CAD build for the part. Positions are in the model's coordinates, mm. Face numbers are marked on the shaded views. Round coordinates to 2 decimals unless told otherwise and drop trailing zeros. Order: outer loops, then holes, each group sorted by start corner. A loop starts at its lowest first (then second) coordinate and runs counter-clockwise, first axis right, second up.
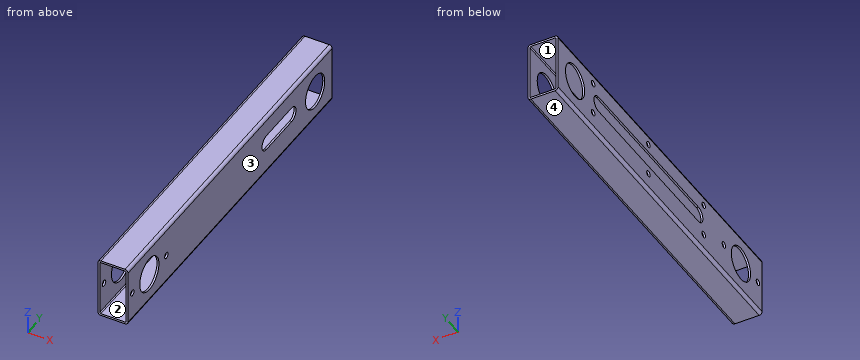
```python
from build123d import *

# Parameters (mm, degrees)
EXTRUDE_THIN1_DEPTH      = 222.25
EXTRUDE_THIN1_DEPTH_BACK = 82.55
CUT_EXTRUDE1_REACH       = 227.134
CUT_EXTRUDE4_REACH       = 227.134
SKETCH4_R                = 2.5527
CUT_EXTRUDE3_DEPTH       = 1.651
SKETCH6_R                = 14.3256
CUT_EXTRUDE5_DEPTH       = 226.134143346
F_10_CLEARANCE_HOLE1_D   = 5.1054


with BuildPart() as part:
    # Sketch1 → Extrude-Thin1 (new, two sides: drawn at the far end of the back side and taken through both)
    with BuildSketch(Plane(origin=(0, 0, 0), x_dir=(1, 0, 0), z_dir=(0, 1, 0)).offset(-EXTRUDE_THIN1_DEPTH_BACK)):
        with BuildLine():
            Line((-10.16, 25.4), (10.16, 25.4))
            ThreePointArc((10.16, 25.4), (11.956051224, 24.656051224), (12.7, 22.86))
            Line((12.7, 22.86), (12.7, -22.86))
            ThreePointArc((12.7, -22.86), (11.956051224, -24.656051224), (10.16, -25.4))
            Line((10.16, -25.4), (-10.16, -25.4))
            ThreePointArc((-10.16, -25.4), (-11.956051224, -24.656051224), (-12.7, -22.86))
            Line((-12.7, -22.86), (-12.7, 22.86))
            ThreePointArc((-12.7, 22.86), (-11.956051224, 24.656051224), (-10.16, 25.4))
        make_face()
        with BuildLine():
            Line((-10.16, 23.749), (10.16, 23.749))
            ThreePointArc((10.16, 23.749), (10.788617928, 23.488617928), (11.049, 22.86))
            Line((11.049, 22.86), (11.049, -22.86))
            ThreePointArc((11.049, -22.86), (10.788617928, -23.488617928), (10.16, -23.749))
            Line((10.16, -23.749), (-10.16, -23.749))
            ThreePointArc((-10.16, -23.749), (-10.788617928, -23.488617928), (-11.049, -22.86))
            Line((-11.049, -22.86), (-11.049, 22.86))
            ThreePointArc((-11.049, 22.86), (-10.788617928, 23.488617928), (-10.16, 23.749))
        make_face(mode=Mode.SUBTRACT)
    extrude(amount=EXTRUDE_THIN1_DEPTH + EXTRUDE_THIN1_DEPTH_BACK)

    # Sketch2 → Cut-Extrude1 (cut, up to next)
    with BuildSketch(Plane.ZY.offset(12.7), mode=Mode.PRIVATE) as cut_extrude1_sk1:
        with BuildLine():
            Line((9.2075, 161.942613489), (9.2075, 12.7))
            ThreePointArc((9.2075, 12.7), (2.54, 6.0325), (-4.1275, 12.7))
            Line((-4.1275, 12.7), (-4.1275, 161.942613489))
            ThreePointArc((-4.1275, 161.942613489), (2.54, 168.610113489), (9.2075, 161.942613489))
        make_face()
    cut_extrude1_tool1 = extrude(cut_extrude1_sk1.sketch, amount=-CUT_EXTRUDE1_REACH, mode=Mode.PRIVATE) & part.part
    add(cut_extrude1_tool1.solids().sort_by_distance((-12.7, 87.321307, 2.54))[0], mode=Mode.SUBTRACT)

    # Sketch5 → Cut-Extrude4 (cut, up to next)
    with BuildSketch(Plane(origin=(12.7, 0, 0), x_dir=(0, 0, -1), z_dir=(1, 0, 0)), mode=Mode.PRIVATE) as cut_extrude4_sk1:
        with BuildLine():
            Line((3.81, 161.942613489), (3.81, 123.842613489))
            ThreePointArc((3.81, 123.842613489), (-2.54, 117.492613489), (-8.89, 123.842613489))
            Line((-8.89, 123.842613489), (-8.89, 161.942613489))
            ThreePointArc((-8.89, 161.942613489), (-2.54, 168.292613489), (3.81, 161.942613489))
        make_face()
    cut_extrude4_tool1 = extrude(cut_extrude4_sk1.sketch, amount=-CUT_EXTRUDE4_REACH, mode=Mode.PRIVATE) & part.part
    add(cut_extrude4_tool1.solids().sort_by_distance((12.7, 142.892613, 2.54))[0], mode=Mode.SUBTRACT)

    # Sketch4 → Cut-Extrude3 (cut)
    with BuildSketch(Plane(origin=(-12.7, 0, 0), x_dir=(0, 0, -1), z_dir=(1, 0, 0))):
        with Locations(Location((11.049, 4.771306688, 0), (0, 0, 180))):
            Circle(SKETCH4_R)
        with Locations(Location((-16.129, 4.771306688, 0), (0, 0, 180))):
            Circle(SKETCH4_R)
        with Locations(Location((-16.129, 87.321306688, 0), (0, 0, 180))):
            Circle(SKETCH4_R)
        with Locations(Location((11.049, 87.321306688, 0), (0, 0, 180))):
            Circle(SKETCH4_R)
        with Locations(Location((-16.129, 169.871306688, 0), (0, 0, 180))):
            Circle(SKETCH4_R)
        with Locations(Location((11.049, 169.871306688, 0), (0, 0, 180))):
            Circle(SKETCH4_R)
    extrude(amount=CUT_EXTRUDE3_DEPTH, mode=Mode.SUBTRACT)

    # Sketch6 → Cut-Extrude5 (cut, through all)
    with BuildSketch(Plane(origin=(12.7, 0, 0), x_dir=(0, 0, -1), z_dir=(1, 0, 0))):
        with Locations((0, -50.8)):
            Circle(SKETCH6_R)
        with Locations((0, 196.85)):
            Circle(SKETCH6_R)
    extrude(amount=-CUT_EXTRUDE5_DEPTH, mode=Mode.SUBTRACT)

    # #10 Clearance Hole1 (through all)
    with Locations(Plane(origin=(12.7, 0, 0), x_dir=(0, 0, -1), z_dir=(1, 0, 0))):
        with Locations((0, -25.4), (0, -76.2)):
            Hole(F_10_CLEARANCE_HOLE1_D / 2)


solid = part.part
```
1. Cut at A-A, the plane y = 196.85. Write the cut outline in (x, z), and give its area (3 significant figures).
2. Pin check, flat tips, straight feed: P1, Ø2, axis at x = 9.5, z = -5, coming from the -Y side; P2, Ø0.8, axis at x = 11.5, y = 147.5, coming from the -Z side; P3, Ø1.3, axis at x = -11.5, y = 87, coming from the +Z side; P4, Ø4.5, axis at y = 4.77, z = 16.13, coming from the -X side. Stop position of each tip, or through.
3. Mould opens along Z. For the marked faces 1, 2, 3 and 4 say: released by +Z, released by -Z, zero draft, split by the parting line, or undercut.
4. Cut at C-C, the plane y = 70. Write the cut outline in (x, z).
5. Cut at B-B, the plane x = -1.25. Write the cut outline in (y, z).
6. Cut at D-D, the plane y = -76.2. Write the cut outline in (x, z).
7. Drill centre lines: line 1 (X direction, y = -60, z = 13); line 2 (Z direction, x = 4.25, y = 188); line 3 (X direction, y = 12, z = -4). Where is each one in solid material? Low to high.
Outcome:
1. outline: (-12.7, -22.86) arc R2.54 ccw to (-10.16, -25.4) - (10.16, -25.4) arc R2.54 ccw to (12.7, -22.86) - (12.7, -14.33) - (11.05, -14.33) - (11.05, -22.86) arc R0.89 cw to (10.16, -23.75) - (-10.16, -23.75) arc R0.89 cw to (-11.05, -22.86) - (-11.05, -14.33) - (-12.7, -14.33) - close; (-12.7, 14.33) - (-11.05, 14.33) - (-11.05, 22.86) arc R0.89 cw to (-10.16, 23.75) - (10.16, 23.75) arc R0.89 cw to (11.05, 22.86) - (11.05, 14.33) - (12.7, 14.33) - (12.7, 22.86) arc R2.54 ccw to (10.16, 25.4) - (-10.16, 25.4) arc R2.54 ccw to (-12.7, 22.86) - close
1. area: 141 mm2
2. P1: passes through
2. P2: stops at z = -25.22
2. P3: stops at z = 25.3
2. P4: stops at x = 11.05
3. face 1: undercut
3. face 2: undercut
3. face 3: zero draft
3. face 4: released by -Z
4. outline: (-12.7, -22.86) arc R2.54 ccw to (-10.16, -25.4) - (10.16, -25.4) arc R2.54 ccw to (12.7, -22.86) - (12.7, 22.86) arc R2.54 ccw to (10.16, 25.4) - (-10.16, 25.4) arc R2.54 ccw to (-12.7, 22.86) - (-12.7, 9.21) - (-11.05, 9.21) - (-11.05, 22.86) arc R0.89 cw to (-10.16, 23.75) - (10.16, 23.75) arc R0.89 cw to (11.05, 22.86) - (11.05, -22.86) arc R0.89 cw to (10.16, -23.75) - (-10.16, -23.75) arc R0.89 cw to (-11.05, -22.86) - (-11.05, -4.13) - (-12.7, -4.13) - close
5. outline: (-82.55, -25.4) - (222.25, -25.4) - (222.25, -23.75) - (-82.55, -23.75) - close; (-82.55, 23.75) - (222.25, 23.75) - (222.25, 25.4) - (-82.55, 25.4) - close
6. outline: (-12.7, -22.86) arc R2.54 ccw to (-10.16, -25.4) - (10.16, -25.4) arc R2.54 ccw to (12.7, -22.86) - (12.7, -2.55) - (11.05, -2.55) - (11.05, -22.86) arc R0.89 cw to (10.16, -23.75) - (-10.16, -23.75) arc R0.89 cw to (-11.05, -22.86) - (-11.05, -2.55) - (-12.7, -2.55) - close; (-12.7, 2.55) - (-11.05, 2.55) - (-11.05, 22.86) arc R0.89 cw to (-10.16, 23.75) - (10.16, 23.75) arc R0.89 cw to (11.05, 22.86) - (11.05, 2.55) - (12.7, 2.55) - (12.7, 22.86) arc R2.54 ccw to (10.16, 25.4) - (-10.16, 25.4) arc R2.54 ccw to (-12.7, 22.86) - close
7. line 1: x = -12.7 to -11.05, 11.05 to 12.7
7. line 2: z = -25.4 to -23.75, 23.75 to 25.4
7. line 3: x = 11.05 to 12.7
